from build123d import *

# Parameters (mm, degrees)
PAD003_DEPTH    = 5
PAD_DEPTH       = 15
SKETCH001_W     = 60
SKETCH001_H     = 15
PAD001_DEPTH    = 65
POCKET_DEPTH    = 15.001
PAD002_DEPTH    = 35
SKETCH004_R     = 15
POCKET001_DEPTH = 103.285271


with BuildPart() as pad003:
    # Sketch005 → Pad003 (new body, symmetric)
    with BuildSketch(Plane.YZ):
        Polygon((0, 0), (-35, 51), (0, 51), align=None)
    extrude(amount=PAD003_DEPTH, both=True)


with BuildPart() as fusion:
    # Sketch → Pad (new body)
    with BuildSketch(Plane.XY):
        with BuildLine():
            ThreePointArc((30, 75), (0, 105), (-30, 75))
            Line((-30, 0), (-30, 75))
            Line((-30, 0), (30, 0))
            Line((30, 0), (30, 75))
        make_face()
    extrude(amount=PAD_DEPTH)

    # Sketch001 → Pad001 (new body)
    with BuildSketch(Plane.XY.offset(15)):
        with Locations((0, 7.5)):
            Rectangle(SKETCH001_W, SKETCH001_H)
    extrude(amount=PAD001_DEPTH)

    # Sketch002 → Pocket (cut, through all)
    with BuildSketch(Plane.XY.offset(15)):
        with BuildLine():
            ThreePointArc((-10, 75.000024), (0, 65), (10, 75.000024))
            Line((10, 109.698372), (10, 75.000024))
            Line((-10, 109.698372), (10, 109.698372))
            Line((-10, 75.000024), (-10, 109.698372))
        make_face()
    extrude(amount=-POCKET_DEPTH, mode=Mode.SUBTRACT)

    # Sketch003 → Pad002 (new body)
    with BuildSketch(Plane.XZ):
        with BuildLine():
            ThreePointArc((-30, 80), (0, 49.999953), (30, 80))
            Line((15, 80), (30, 80))
            ThreePointArc((-15, 80), (0, 64.999953), (15, 80))
            Line((-15, 80), (-30, 80))
        make_face()
    extrude(amount=PAD002_DEPTH)

    # Sketch004 → Pocket001 (cut, through all)
    with BuildSketch(Plane.XZ):
        with Locations((0, 79.999953)):
            Circle(SKETCH004_R)
    extrude(amount=-POCKET001_DEPTH, mode=Mode.SUBTRACT)

    # Fusion: union Pad003
    add(pad003.part)


solid = fusion.part
The listing builds one solid part. Answer for the finished solid, in the listing's coordinates (mm). A direction names the side the tool comes from. Give positions to 0.01 mm unless a question says otherwise; leave off trailing zeros. Write each loop counter-clockwise with the first axis right and the second up, starting at its lowest first coordinate (ties: lowest second). Pieces come first, ordered by that corner, then holes. Notation, with made-up numbers: (30, -20.75) - (81, -20.75) arc R27 ccw to (81, 16.25) - close; hole circle Ø6 at (76.25, -38). An arc over 180 degrees is marked (long way). One line per question, with ' | ' between items. Start each with the question number.
1. Section C-C, the plane y = 35 is taken. Determine the outline of the cut face in (x, z), then the cut area to 3 significant figures.
2. Section A-A, the plane y = -14 is taken. Determine the outline of the cut face in (x, z), then the cut area to 3 significant figures.
3. Section B-B, the plane z = 63 is taken. Determine the outline of the cut face in (x, y), then the cut area to 3 significant figures.
4. For faces 5 (the face through (0, 50, 15)), 6 (the face through (-5, -13, 31)), 7 (the face through (-22, -10, 80)), 8 (the face through (17, 0, 31)), determine the directions among +Z, -Z, +X, -X, +Y, -Y from which every point of the face is accessible in a straight line to the end or side of a thin tool.
5. Straight lines are drawn through the part: line 1 (Z direction, x = -19, y = 27); line 2 (Y direction, x = -6, z = 58). For each, find the intervals that lie inside material, in ascending order.
6. Determine the mould class of faces 1 (the face through (10, 89, 8)), 2 (the face through (-10, 89, 8)), 3 (the face through (-10.878, -17.255, 52.042)), 4 (the face through (0, -35, 62)) for opening direction X: +X half, -X half, draft (parallel to the pull), parting line (faces both ways), or undercut.
7. Given P1, Ø10, axis at x = 1.5, y = -7, coming from the -Z side; P2, Ø18, axis at x = 3, z = 46.5, coming from the +Y side; P3, Ø12, axis at y = 89.5, z = 5, coming from the -X side, each flat-ended and moving along its own axis, determine where each tip first touches the part or whether it passes through.
Result:
1) outline: (-30, 0) - (30, 0) - (30, 15) - (-30, 15) - close | area: 900 mm2
2) outline: (-30, 80) arc R30 ccw to (-5, 50.42) - (-5, 20.4) - (5, 20.4) - (5, 50.42) arc R30 ccw to (30, 80) - (15, 80) arc R15 cw to (-15, 80) - close | area: 1,360 mm2
3) outline: (-30, 0) - (-24.72, 0) - (-24.72, -35) - (24.72, -35) - (24.72, 0) - (30, 0) - (30, 15) - (-30, 15) - close | area: 2,630 mm2
4) face 5: +Z, +X, -X, +Y | face 6: -Z, -X, -Y | face 7: +Z, +X, -X, +Y, -Y | face 8: -Z, +X, -Y
5) line 1: z = 0 to 15 | line 2: y = -35 to 15
6) face 1: undercut | face 2: undercut | face 3: parting line | face 4: draft
7) P1: stops at z = 2.91 | P2: stops at y = 15 | P3: stops at x = -28.77
